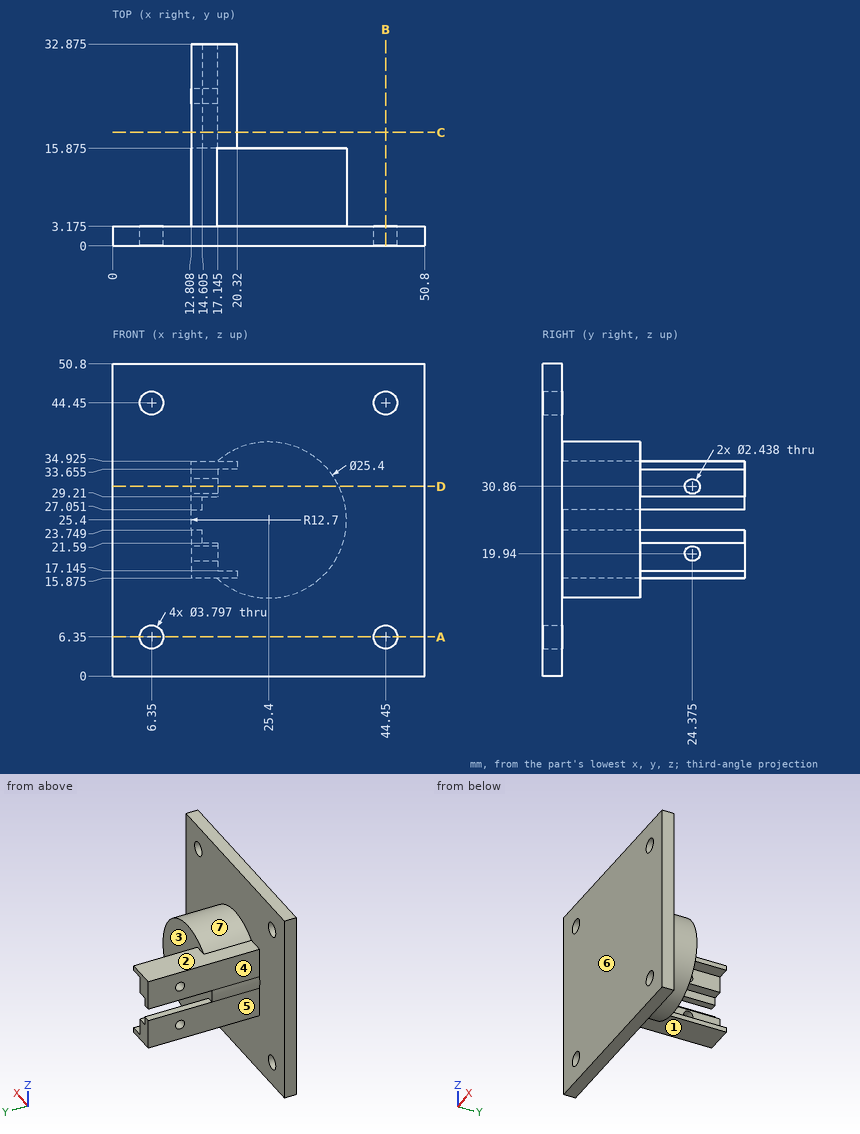
Source: three-view drawing plus pictorial views. Frame: mm from the lowest corner of the part. A direction names the side the tool comes from. Coordinates: 2 decimals unless noted, no trailing zeros. Order: outer loops, then holes, each group sorted by start corner. A loop starts at its lowest first (then second) coordinate and runs counter-clockwise, first axis right, second up.
1) Section D-D (z = 30.86). Return loops of the section in (x, y) (1 decimal).
Result sheet:
outline: (0, 0) - (50.8, 0) - (50.8, 3.2) - (36.9, 3.2) - (36.9, 15.9) - (17.1, 15.9) - (17.1, 23.2) - (12.8, 23.2) - (12.8, 3.2) - (0, 3.2) - close; (12.8, 25.6) - (17.1, 25.6) - (17.1, 32.9) - (12.8, 32.9) - close
2) Set-up query: the marked faces 5, 6 and 7. Return all of +Z, -Z, +X, -X, +Y, -Y with unobstructed straight access to the full face (end or side cutting, diameter ignored); none if empty.
Result sheet:
face 5: -Z, -X, +Y
face 6: +Z, -Z, +X, -X, -Y
face 7: +Y
3) Section A-A (z = 6.35). Return loops of the section in (x, y) (1 decimal).
Result sheet:
outline: (0, 0) - (4.5, 0) - (4.5, 3.2) - (0, 3.2) - close; (8.2, 0) - (42.6, 0) - (42.6, 3.2) - (8.2, 3.2) - close; (46.3, 0) - (50.8, 0) - (50.8, 3.2) - (46.3, 3.2) - close
4) Draft query along Z for the marked faces 1, 2, 3 and 4. Return one class per face: released by +Z, released by -Z, zero draft, split by the parting line, or undercut.
Result sheet:
face 1: released by -Z
face 2: released by +Z
face 3: undercut
face 4: zero draft
5) Ray query, probe 1 along Z at (x, y) = (6.35, 0.7); probe 2 along Z at (x, y) = (17.5, 21.5) (1 decimal). Return the intervals inside material, ascending.
Result sheet:
probe 1: z = 0 to 4.45, 8.25 to 42.55, 46.35 to 50.8
probe 2: z = 15.9 to 17.1, 33.7 to 34.9
6) Section B-B (x = 44.45). Return loops of the section in (y, z) (1 decimal), then the cut area to 3 significant figures.
Result sheet:
outline: (0, 0) - (3.2, 0) - (3.2, 4.5) - (0, 4.5) - close; (0, 8.2) - (3.2, 8.2) - (3.2, 42.6) - (0, 42.6) - close; (0, 46.3) - (3.2, 46.3) - (3.2, 50.8) - (0, 50.8) - close
area: 137 mm2
7) First-contact query: P1, Ø5, axis at x = 6.35, z = 44.45, coming from the -Y side; P2, Ø5, axis at y = 23, z = 31.5, coming from the -X side; P3, Ø6, axis at x = 32, z = 42.5, coming from the +Y side (3 decimals); P4, Ø3.5, axis at y = 22.5, z = 31, coming from the +X side (3 decimals). Flat tips, straight axial feed; report the tip coordinate or a pass-through.
Result sheet:
P1: stops at y = 0
P2: stops at x = 12.81
P3: stops at y = 3.175
P4: stops at x = 17.145
8) Section C-C (y = 18.5). Return loops of the section in (x, z) (1 decimal), then the cut area to 3 significant figures.
Result sheet:
outline: (12.8, 15.9) - (20.3, 15.9) - (20.3, 17.1) - (17.1, 17.1) - (17.1, 21.6) - (14.6, 21.6) - (14.6, 23.7) - (12.8, 23.7) - close; (12.8, 27.1) - (14.6, 27.1) - (14.6, 29.2) - (17.1, 29.2) - (17.1, 33.7) - (20.3, 33.7) - (20.3, 34.9) - (12.8, 34.9) - close
area: 65.4 mm2
